For this review, use the dimensioned drawing (mm, ordinates from the lowest corner) and the shaded views. A direction names the side the tool comes from. Round coordinates to 2 decimals unless told otherwise and drop trailing zeros. Write each loop counter-clockwise with the first axis right and the second up, starting at its lowest first coordinate (ties: lowest second). Pieces come first, ordered by that corner, then holes.
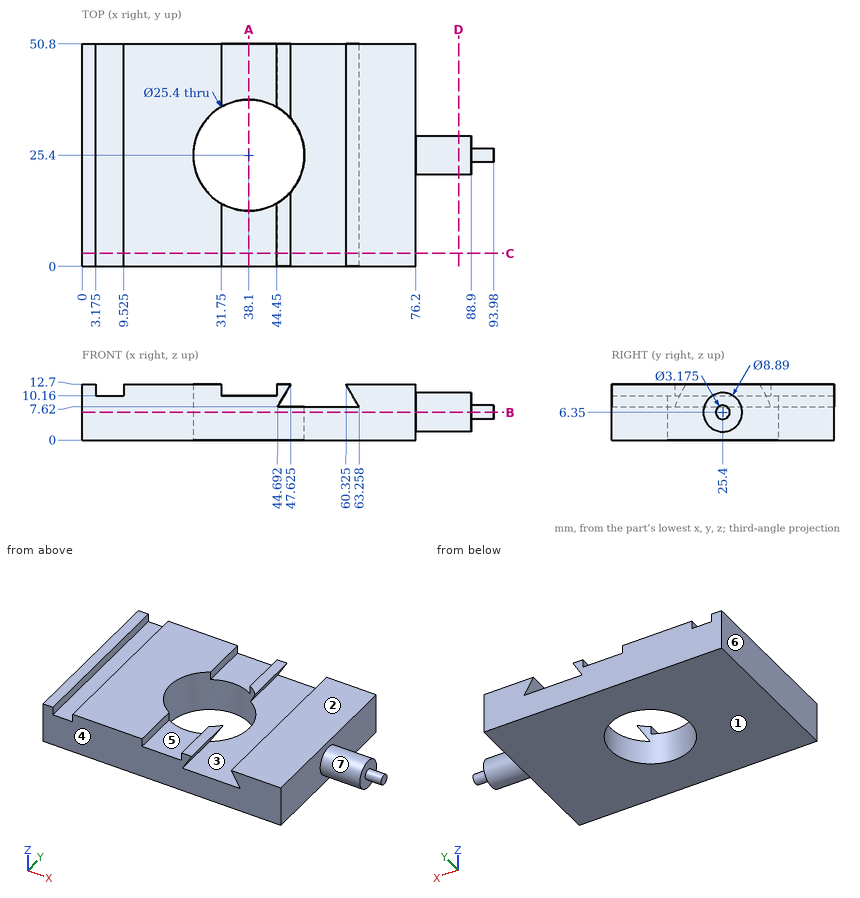
1) For P1, Ø1.5, axis at y = 13.5, z = 6, coming from the +X side; P2, Ø4, axis at x = 37, y = 7, coming from the +Z side, all flat-tipped, find the tip position at first contact; note any pin that passes through.
2) Add section B-B on z = 6.35. State the section outline as (x, y) points (1 decimal).
3) Add section C-C on y = 3. State the section outline as (x, z) points (3 decimals).
4) Add section A-A on x = 38.1. State the section outline as (y, z) points.
5) Add section D-D on x = 86. State the section outline as (y, z) points (3 decimals).
6) For the marked faces 5, 6 and 7, list the 3-axis set-ups (+Z, -Z, +X, -X, +Y, -Y) from which the entire face can be reached by the end or side of a thin tool; tool diameter is ignored.
7) The part is to be moulded in two halves that separate along Z. For the marked faces 1, 2, 3 and 4, say which applies: pulls with the +Z half, pulls with the -Z half, needs draft (parallel to the pull), parting line crosses it, or undercut.
8) For line 1 along Y through (x, z) = (38.1, 7.75); line 2 along X through (y, z) = (48.5, 10.75) (3 decimals); line 3 along X through (y, z) = (29.5, 10.5) (3 decimals), list the stretches that pass through material, from the lowest coordinate up.
Computed:
1. P1: stops at x = 76.2
1. P2: stops at z = 10.16
2. outline: (0, 0) - (76.2, 0) - (76.2, 21) - (88.9, 21) - (88.9, 23.8) - (94, 23.8) - (94, 27) - (88.9, 27) - (88.9, 29.8) - (76.2, 29.8) - (76.2, 50.8) - (0, 50.8) - close; hole circle Ø25.4 at (38.1, 25.4)
3. outline: (0, 0) - (76.2, 0) - (76.2, 12.7) - (60.325, 12.7) - (63.258, 7.62) - (44.692, 7.62) - (47.625, 12.7) - (44.45, 12.7) - (44.45, 10.16) - (31.75, 10.16) - (31.75, 12.7) - (9.525, 12.7) - (9.525, 10.16) - (3.175, 10.16) - (3.175, 12.7) - (0, 12.7) - close
4. outline: (0, 0) - (12.7, 0) - (12.7, 10.16) - (0, 10.16) - close; (38.1, 0) - (50.8, 0) - (50.8, 10.16) - (38.1, 10.16) - close
5. outline: circle Ø8.89 at (25.4, 6.35)
6. face 5: +Z, +Y, -Y
6. face 6: +Z, -Z, -X, +Y, -Y
6. face 7: +X
7. face 1: pulls with the -Z half
7. face 2: pulls with the +Z half
7. face 3: undercut
7. face 4: needs draft
8. line 1: y = 0 to 12.7, 38.1 to 50.8
8. line 2: x = 0 to 3.175, 9.525 to 31.75, 44.45 to 46.499, 61.451 to 76.2
8. line 3: x = 0 to 3.175, 9.525 to 26.08, 61.595 to 76.2
